The model under review builds one solid part; all positions refer to its coordinate system, in mm. Face numbers are marked on the shaded views. Round coordinates to 2 decimals unless told otherwise and drop trailing zeros. Loops run counter-clockwise (first coordinate to the right, second up) from the corner with the lowest first, then second, coordinate; pieces in that order, holes last. Notation, with made-up numbers: (-8, -15) -> (51, -15) arc R20 cw to (51, 0) -> close; hole circle Ø4 at (-20.75, 34.25). An arc over 180 degrees is marked (long way). Use CSV: the item, a comma, the result in double quotes. Start each with the question number.
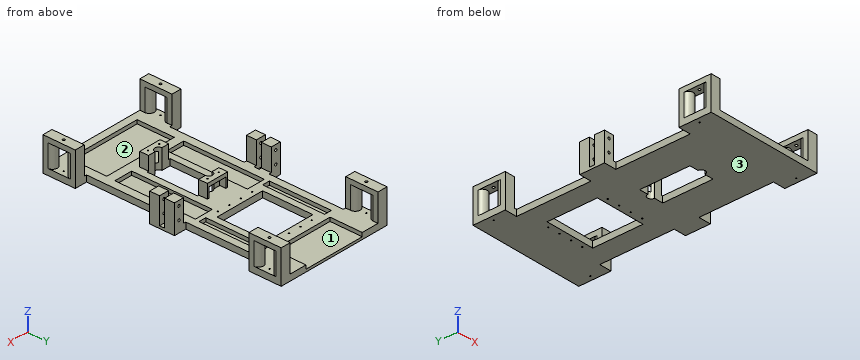
```python
from build123d import *

# Parameters (mm, degrees)
SKETCH_R        = 0.5
SKETCH_W        = 40.5
SKETCH_H        = 40.5
PAD_DEPTH       = 5
SKETCH001_W     = 50
SKETCH001_H     = 29.097618
SKETCH001_W_2   = 6
SKETCH001_H_2   = 50
SKETCH001_W_3   = 21.595833
SKETCH001_H_3   = 4.1
SKETCH001_W_4   = 20.110661
SKETCH001_W_5   = 15
SKETCH001_H_4   = 65
SKETCH001_W_6   = 60
SKETCH001_H_5   = 30
POCKET_DEPTH    = 3
SKETCH002_W     = 8
SKETCH002_H     = 7.95
PAD001_DEPTH    = 18
SKETCH003_R     = 1
POCKET001_DEPTH = 20
PAD002_DEPTH    = 18
SKETCH005_W     = 8
SKETCH005_H     = 26
SKETCH005_R     = 1
PAD003_DEPTH    = 4
SKETCH006_R     = 0.5
PAD004_DEPTH    = 11
SKETCH007_W     = 15
SKETCH007_H     = 8
POCKET002_DEPTH = 5
SKETCH008_W     = 15
SKETCH008_H     = 8
POCKET003_DEPTH = 5


with BuildPart() as part:
    # Sketch → Pad (new body)
    with BuildSketch(Plane.XY):
        Polygon((-47, 96), (47, 96), (47, 70), (37, 70), (37, 10), (47, 10), (47, -10), (37, -10), (37, -70), (47, -70), (47, -96), (-47, -96), (-47, -70), (-37, -70), (-37, -10), (-47, -10), (-47, 10), (-37, 10), (-37, 70), (-47, 70), align=None)
        with Locations((-15.1, 64.25)):
            Circle(SKETCH_R, mode=Mode.SUBTRACT)
        with Locations((-5.1, 64.25)):
            Circle(SKETCH_R, mode=Mode.SUBTRACT)
        with Locations((5.1, 64.25)):
            Circle(SKETCH_R, mode=Mode.SUBTRACT)
        with Locations((15.1, 64.25)):
            Circle(SKETCH_R, mode=Mode.SUBTRACT)
        with Locations((-15.1, 16.25)):
            Circle(SKETCH_R, mode=Mode.SUBTRACT)
        with Locations((-5.1, 16.25)):
            Circle(SKETCH_R, mode=Mode.SUBTRACT)
        with Locations((5.1, 16.25)):
            Circle(SKETCH_R, mode=Mode.SUBTRACT)
        with Locations((15.1, 16)):
            Circle(SKETCH_R, mode=Mode.SUBTRACT)
        with Locations((-43, 83)):
            Circle(SKETCH_R, mode=Mode.SUBTRACT)
        with Locations((43, 83)):
            Circle(SKETCH_R, mode=Mode.SUBTRACT)
        with Locations((43, -83)):
            Circle(SKETCH_R, mode=Mode.SUBTRACT)
        with Locations((-43, -83)):
            Circle(SKETCH_R, mode=Mode.SUBTRACT)
        with Locations((0, 40.25)):
            Rectangle(SKETCH_W, SKETCH_H, mode=Mode.SUBTRACT)
        with BuildLine():
            Line((-10.25, -5), (-3, -5))
            ThreePointArc((3, -5), (0, -2), (-3, -5))
            Line((3, -5), (10.25, -5))
            Line((10.25, -5), (10.25, -45.5))
            Line((10.25, -45.5), (3, -45.5))
            ThreePointArc((-3, -45.5), (0, -48.5), (3, -45.5))
            Line((-3, -45.5), (-10.25, -45.5))
            Line((-10.25, -45.5), (-10.25, -5))
        make_face(mode=Mode.SUBTRACT)
    extrude(amount=PAD_DEPTH)

    # Sketch001 → Pocket (cut)
    with BuildSketch(Plane.XY.offset(5)):
        with Locations((0, 84.548809)):
            Rectangle(SKETCH001_W, SKETCH001_H)
        with Locations((-28.241235, 40.47918)):
            Rectangle(SKETCH001_W_2, SKETCH001_H_2)
        with Locations((28.241235, 40.47918)):
            Rectangle(SKETCH001_W_2, SKETCH001_H_2)
        with Locations((-47.797916, 0)):
            Rectangle(SKETCH001_W_3, SKETCH001_H_3)
        with Locations((47.05533, 0)):
            Rectangle(SKETCH001_W_4, SKETCH001_H_3)
        with Locations((-23.110925, -20.5)):
            Rectangle(SKETCH001_W_5, SKETCH001_H_4)
        with Locations((23.110925, -20.5)):
            Rectangle(SKETCH001_W_5, SKETCH001_H_4)
        with Locations((0, -75)):
            Rectangle(SKETCH001_W_6, SKETCH001_H_5)
    extrude(amount=-POCKET_DEPTH, mode=Mode.SUBTRACT)

    # Sketch002 → Pad001 (new body)
    with BuildSketch(Plane.XY.offset(5)):
        with Locations((43, 6.025)):
            Rectangle(SKETCH002_W, SKETCH002_H)
        with Locations((43, -6.025)):
            Rectangle(SKETCH002_W, SKETCH002_H)
    pad001 = extrude(amount=PAD001_DEPTH)

    # Mirrored: Pad001 across Sketch002 V_Axis
    add(pad001.mirror(Plane(origin=(0, 0, 5), x_dir=(0, 0, 1), z_dir=(1, 0, 0))))

    # Sketch003 → Pocket001 (cut)
    with BuildSketch(Plane.XZ.offset(10)):
        with Locations((43, 19)):
            Circle(SKETCH003_R)
        with Locations((43, 9)):
            Circle(SKETCH003_R)
    pocket001 = extrude(amount=-POCKET001_DEPTH, mode=Mode.SUBTRACT)

    # Mirrored001: Pocket001 across Sketch003 V_Axis
    add(pocket001.mirror(Plane(origin=(0, -10, 0), x_dir=(0, -1, 0), z_dir=(1, 0, 0))), mode=Mode.SUBTRACT)

    # Sketch004 → Pad002 (new body)
    with BuildSketch(Plane.XY.offset(5)):
        with BuildLine():
            Line((39, 96), (47, 96))
            Line((47, 96), (47, 92))
            ThreePointArc((39, 92), (43, 88), (47, 92))
            Line((39, 92), (39, 96))
        make_face()
        with BuildLine():
            Line((47, 74.000025), (47, 70))
            Line((47, 70), (39, 70))
            Line((39, 70), (39, 74))
            ThreePointArc((47, 74.000025), (42.999988, 78.000012), (39, 74))
        make_face()
        with BuildLine():
            Line((39, -70), (47, -70))
            Line((47, -70), (47, -74))
            ThreePointArc((39, -74), (43, -78), (47, -74))
            Line((39, -74), (39, -70))
        make_face()
        with BuildLine():
            Line((47, -92), (47, -96))
            Line((47, -96), (39, -96))
            Line((39, -96), (39, -92))
            ThreePointArc((47, -92), (43, -88), (39, -92))
        make_face()
    pad002 = extrude(amount=PAD002_DEPTH)

    # Mirrored002: Pad002 across Sketch004 V_Axis
    add(pad002.mirror(Plane(origin=(0, 0, 5), x_dir=(0, 0, 1), z_dir=(1, 0, 0))))

    # Sketch005 → Pad003 (new body)
    with BuildSketch(Plane.XY.offset(23)):
        with Locations((43, 83)):
            Rectangle(SKETCH005_W, SKETCH005_H)
        with Locations((43, 83)):
            Circle(SKETCH005_R, mode=Mode.SUBTRACT)
        with Locations((43, -83)):
            Rectangle(SKETCH005_W, SKETCH005_H)
        with Locations((43, -83)):
            Circle(SKETCH005_R, mode=Mode.SUBTRACT)
    pad003 = extrude(amount=PAD003_DEPTH)

    # Mirrored003: Pad003 across Sketch005 V_Axis
    add(pad003.mirror(Plane(origin=(0, 0, 23), x_dir=(0, 0, 1), z_dir=(1, 0, 0))))

    # Sketch006 → Pad004 (new body)
    with BuildSketch(Plane.XY.offset(5)):
        with BuildLine():
            Line((-9, 2), (9, 2))
            Line((9, 2), (9, -5))
            Line((9, -5), (3, -5))
            ThreePointArc((3, -5), (0, -2), (-3, -5))
            Line((-3, -5), (-9, -5))
            Line((-9, -5), (-9, 2))
        make_face()
        with Locations((-5, -1.5)):
            Circle(SKETCH006_R, mode=Mode.SUBTRACT)
        with Locations((5, -1.5)):
            Circle(SKETCH006_R, mode=Mode.SUBTRACT)
        with BuildLine():
            Line((-9, -45.5), (-3, -45.5))
            ThreePointArc((-3, -45.5), (0, -48.5), (3, -45.5))
            Line((3, -45.5), (9, -45.5))
            Line((9, -45.5), (9, -52.5))
            Line((9, -52.5), (-9, -52.5))
            Line((-9, -52.5), (-9, -45.5))
        make_face()
        with Locations((-5, -49.5)):
            Circle(SKETCH006_R, mode=Mode.SUBTRACT)
        with Locations((5, -49.5)):
            Circle(SKETCH006_R, mode=Mode.SUBTRACT)
    extrude(amount=PAD004_DEPTH)

    # Sketch007 → Pocket002 (cut)
    with BuildSketch(Plane.XZ.offset(52.5)):
        with Locations((0, 9)):
            Rectangle(SKETCH007_W, SKETCH007_H)
    extrude(amount=-POCKET002_DEPTH, mode=Mode.SUBTRACT)

    # Sketch008 → Pocket003 (cut)
    with BuildSketch(Plane(origin=(0, 2, 0), x_dir=(-1, 0, 0), z_dir=(0, 1, 0))):
        with Locations((0, 9)):
            Rectangle(SKETCH008_W, SKETCH008_H)
    extrude(amount=-POCKET003_DEPTH, mode=Mode.SUBTRACT)


solid = part.part
```
1. For line 1 along Y through (x, z) = (43, 25.2); line 2 along X through (y, z) = (83, 1.85); line 3 along Y through (x, z) = (-4, 3), list the stretches that pass through material, from the lowest coordinate up. Write a range as from..to.
2. Clearance check with flat-ended pins moving along their axes: P1, Ø4, axis at y = -31, z = 2, coming from the +X side; P2, Ø2.5, axis at x = 5.5, z = 8, coming from the +Y side; P3, Ø1.6, axis at x = 43, y = -83, coming from the +Z side; P4, Ø1, axis at y = 74.5, z = 10, coming from the +X side. State where each tip first meets the part, or that it passes through.
3. Take a section at A-A, the plane y = 34. Give the boundary of the cut face in (x, z), then the cut area to 4 significant figures.
4. The part is to be moulded in two halves that separate along X. For the marked faces 1, 2 and 3, say which applies: pulls with the +X half, pulls with the -X half, needs draft (parallel to the pull), parting line crosses it, or undercut.
5. Take a section at B-B, the plane y = -64. Give the boundary of the cut face in (x, z), then the cut area to 3 significant figures.
Results:
1,line 1,"-96..-84, -82..-70, 70..82, 84..96"
1,line 2,"-47..-43.5, -42.5..42.5, 43.5..47"
1,line 3,"-96..-90, -60..-45.5, -5..20, 60.5..70"
2,P1,"x = 37"
2,P2,"y = -3"
2,P3,"z = 5"
2,P4,"x = 47"
3,outline,"(-37, 0) -> (-20.25, 0) -> (-20.25, 5) -> (-25.24, 5) -> (-25.24, 2) -> (-31.24, 2) -> (-31.24, 5) -> (-37, 5) -> close; (20.25, 0) -> (37, 0) -> (37, 5) -> (31.24, 5) -> (31.24, 2) -> (25.24, 2) -> (25.24, 5) -> (20.25, 5) -> close"
3,area,"131.5 mm²"
4,face 1,"undercut"
4,face 2,"undercut"
4,face 3,"needs draft"
5,outline,"(-37, 0) -> (37, 0) -> (37, 5) -> (30, 5) -> (30, 2) -> (-30, 2) -> (-30, 5) -> (-37, 5) -> close"
5,area,"190 mm²"
